Work out the finished part from the listing and answer in its coordinate system (mm). Face numbers are marked on the shaded views. A direction names the side the tool comes from. Round coordinates to 2 decimals unless told otherwise and drop trailing zeros. Loops run counter-clockwise (first coordinate to the right, second up) from the corner with the lowest first, then second, coordinate; pieces in that order, holes last. Notation, with made-up numbers: (67, -12.5) - (91, -12.5) arc R6 ccw to (91, -4.5) - close; hole circle Ø1 at (39, 32.25). An arc over 180 degrees is marked (long way). Return JSON: item names as keys, results as strings.
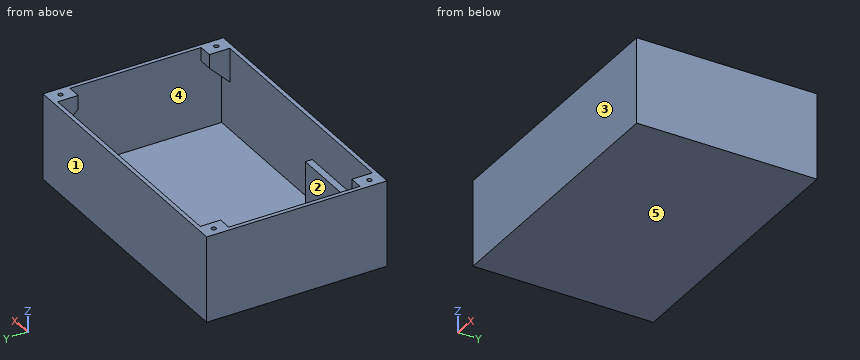
Autodesk Inventor part; units mm, degrees
ref_plane "YZ Plane" through (0, 0, 0) normal (1, 0, 0) x (0, 1, 0)
ref_plane "XZ Plane" through (0, 0, 0) normal (0, 1, 0) x (-1, 0, 0)
ref_plane "XY Plane" through (0, 0, 0) normal (0, 0, 1) x (1, 0, 0)
sketch "Sketch7" plane through (0, 0, 0) normal (0, 0, 1) x (1, 0, 0)
  line L0 (100.625, -66.125) -> (-100.625, -66.125)
  line L1 (-100.625, -66.125) -> (-100.625, 66.125)
  line L2 (-100.625, 66.125) -> (100.625, 66.125)
  line L3 (100.625, 66.125) -> (100.625, -66.125)
  line L4 (100.625, -66.125) -> (-100.625, 66.125) construction
  line L5 (-100.625, -66.125) -> (100.625, 66.125) construction
  point P0 (0, 0)
  dimension "d15" = 201.25
  dimension "d16" = 132.25
extrude "Box Outside" add sketch "Sketch7" along normal blind 63
sketch "Sketch8" plane through (0, 0, 63) normal (0, 0, 1) x (1, 0, 0)
  line L0 (-97.625, 63.125) -> (97.625, 63.125)
  line L1 (97.625, 63.125) -> (97.625, -63.125)
  line L2 (97.625, -63.125) -> (-97.625, -63.125)
  line L3 (-97.625, -63.125) -> (-97.625, 63.125)
  line L4 (100.625, 66.125) -> (-100.625, 66.125)
  line L5 (-100.625, 66.125) -> (-100.625, -66.125)
  line L6 (-100.625, -66.125) -> (100.625, -66.125)
  line L7 (100.625, -66.125) -> (100.625, 66.125)
  point P0 (0, 0)
  dimension "d19" = 3
  dimension "d20" = 3
  dimension "d21" = 3
  dimension "d22" = 3
extrude "Box Cut" cut sketch "Sketch8" against normal blind 60 contours L0 L1 L2 L3
sketch "Sketch9" plane through (-97.625, -63.125, 63) normal (0, 1, 0) x (1, 0, 0)
  line L0 (0, 0) -> (10, 0)
  line L1 (10, 0) -> (10, 25)
  line L2 (10, 25) -> (0, 25)
  line L3 (0, 25) -> (0, 0)
  point P0 (97.625, 63)
  dimension "d25" = 10
  dimension "d26" = 25
extrude "ScrewHole Box LB" add sketch "Sketch9" along normal blind 15
sketch "Sketch10" plane through (-97.625, -63.125, 3) normal (0, 1, 0) x (1, 0, 0)
  line L0 (195.25, -60) -> (195.25, 0)
  line L1 (195.25, -60) -> (185.25, -60)
  line L2 (185.25, -60) -> (185.25, -35)
  line L3 (185.25, -35) -> (195.25, -35)
  line L4 (195.25, -35) -> (195.25, -60)
  point P0 (97.625, 3)
  dimension "d29" = 10
  dimension "d30" = 25
extrude "ScrewHole Box RB" add sketch "Sketch10" along normal blind 15
sketch "Sketch11" plane through (-97.625, 63.125, 63) normal (0, -1, 0) x (1, 0, 0)
  line L0 (0, 0) -> (195.25, 0)
  line L1 (0, 0) -> (10, 0)
  line L2 (10, 0) -> (10, -25)
  line L3 (10, -25) -> (0, -25)
  line L4 (0, -25) -> (0, 0)
  point P0 (97.625, -63)
  dimension "d33" = 10
  dimension "d34" = 25
extrude "ScrewHole Box LU" add sketch "Sketch11" along normal blind 15
sketch "Sketch13" plane through (97.625, -63.125, 3) normal (-1, 0, 0) x (0, 0, 1)
  line L0 (60, 126.25) -> (0, 126.25)
  line L1 (60, 126.25) -> (35, 126.25)
  line L2 (35, 126.25) -> (35, 111.25)
  line L3 (35, 111.25) -> (60, 111.25)
  line L4 (60, 111.25) -> (60, 126.25)
  point P0 (-3, 63.125)
  dimension "d37" = 25
  dimension "d38" = 15
extrude "ScrewHole Box RU" add sketch "Sketch13" along normal blind 10
sketch "Sketch27" plane through (0, 0, 63) normal (0, 0, 1) x (1, 0, 0)
  line L0 (-87.625, -63.125) -> (-87.625, -48.125)
  line L1 (-100.625, 66.125) -> (-100.625, -66.125)
  line L2 (-87.625, -48.125) -> (-100.625, -48.125)
  line L3 (-100.625, -48.125) -> (-100.625, -66.125)
  line L4 (-100.625, -66.125) -> (-87.625, -66.125)
  line L5 (-87.625, -66.125) -> (-87.625, -48.125)
  line L6 (-87.625, -48.125) -> (-100.625, -66.125)
  line L7 (-87.625, -66.125) -> (-100.625, -48.125)
  circle A0 centre (-94.125, -57.125) radius 2.4
  point P0 (0, 0)
  dimension "d84" = 4.8
extrude "Outside ScrewHole LB" cut sketch "Sketch27" against normal blind 26 contours A0 L7 L6 | L6 L7 A0 | A0 L6 L7 | L7 L6 A0
sketch "Sketch29" plane through (0, 0, 63) normal (0, 0, 1) x (1, 0, 0)
  line L0 (-87.625, -63.125) -> (-87.625, -48.125)
  line L1 (-100.625, -66.125) -> (100.625, -66.125)
  line L2 (-87.625, -48.125) -> (-100.625, -48.125)
  line L3 (-100.625, -48.125) -> (-100.625, -66.125)
  line L4 (-100.625, -66.125) -> (-87.625, -66.125)
  line L5 (-87.625, -66.125) -> (-87.625, -48.125)
  line L6 (-87.625, -48.125) -> (-100.625, -66.125)
  circle A0 centre (-94.125, -57.125) radius 2.4
  point P0 (0, 0)
extrude "ScrewRibbon LB" add sketch "Sketch29" against normal blind 2 contours A0 L6 | L6 A0
sketch "Sketch30" plane through (0, 0, 63) normal (0, 0, 1) x (1, 0, 0)
  line L0 (-97.625, -48.125) -> (-87.625, -48.125)
  line L1 (-100.625, -66.125) -> (100.625, -66.125)
  line L2 (-87.625, -48.125) -> (-100.625, -48.125)
  line L3 (-100.625, -48.125) -> (-100.625, -66.125)
  line L4 (-100.625, -66.125) -> (-87.625, -66.125)
  line L5 (-87.625, -66.125) -> (-87.625, -48.125)
  line L6 (-87.625, -48.125) -> (-100.625, -66.125)
  circle A0 centre (-94.125, -57.125) radius 1.7
  point P0 (0, 0)
  dimension "d92" = 3.4
extrude "Inside ScrewHole LB" cut sketch "Sketch30" against normal blind 24 contours A0 L6 | L6 A0
sketch "Sketch31" plane through (0, 0, 63) normal (0, 0, 1) x (1, 0, 0)
  line L0 (-100.625, 66.125) -> (-100.625, -66.125)
  line L1 (-87.625, 48.125) -> (-97.625, 48.125)
  line L2 (-100.625, 66.125) -> (-87.625, 66.125)
  line L3 (-87.625, 66.125) -> (-87.625, 48.125)
  line L4 (-87.625, 48.125) -> (-100.625, 48.125)
  line L5 (-100.625, 48.125) -> (-100.625, 66.125)
  line L6 (-100.625, 66.125) -> (-87.625, 48.125)
  circle A0 centre (-94.125, 57.125) radius 2.4
  point P0 (0, 0)
  dimension "d95" = 4.8
extrude "Outside ScrewHole LU" cut sketch "Sketch31" against normal blind 24 contours A0 L6 | L6 A0
sketch "Sketch32" plane through (0, 0, 63) normal (0, 0, 1) x (1, 0, 0)
  line L0 (-97.625, 48.125) -> (-87.625, 48.125)
  line L1 (-100.625, 66.125) -> (-100.625, -66.125)
  line L2 (-87.625, 48.125) -> (-100.625, 48.125)
  line L3 (-100.625, 48.125) -> (-100.625, 66.125)
  line L4 (-100.625, 66.125) -> (-87.625, 66.125)
  line L5 (-87.625, 66.125) -> (-87.625, 48.125)
  line L6 (-87.625, 66.125) -> (-100.625, 48.125)
  circle A0 centre (-94.125, 57.125) radius 2.4
  point P0 (0, 0)
  dimension "d98" = 4.8
extrude "ScrewRibbon LU" add sketch "Sketch32" against normal blind 2 contours A0 L6 | L6 A0
sketch "Sketch33" plane through (0, 0, 63) normal (0, 0, 1) x (1, 0, 0)
  line L0 (100.625, 66.125) -> (-100.625, 66.125)
  line L1 (-87.625, 48.125) -> (-97.625, 48.125)
  line L2 (-100.625, 66.125) -> (-87.625, 66.125)
  line L3 (-87.625, 66.125) -> (-87.625, 48.125)
  line L4 (-87.625, 48.125) -> (-100.625, 48.125)
  line L5 (-100.625, 48.125) -> (-100.625, 66.125)
  line L6 (-100.625, 66.125) -> (-87.625, 48.125)
  circle A0 centre (-94.125, 57.125) radius 1.7
  point P0 (0, 0)
  dimension "d101" = 3.4
extrude "Inside ScrewHole LU" cut sketch "Sketch33" against normal blind 21.75 contours A0 L6 | L6 A0
sketch "Sketch34" plane through (0, 0, 63) normal (0, 0, 1) x (1, 0, 0)
  line L0 (87.625, 48.125) -> (87.625, 63.125)
  line L1 (100.625, 66.125) -> (-100.625, 66.125)
  line L2 (87.625, 48.125) -> (100.625, 48.125)
  line L3 (100.625, 48.125) -> (100.625, 66.125)
  line L4 (100.625, 66.125) -> (87.625, 66.125)
  line L5 (87.625, 66.125) -> (87.625, 48.125)
  line L6 (100.625, 66.125) -> (87.625, 48.125)
  circle A0 centre (94.125, 57.125) radius 2.4
  point P0 (0, 0)
  dimension "d104" = 4.8
extrude "Outside ScrewHole RU" cut sketch "Sketch34" against normal blind 37 contours A0 L6 | L6 A0
sketch "Sketch35" plane through (0, 0, 63) normal (0, 0, 1) x (1, 0, 0)
  line L0 (100.625, -66.125) -> (100.625, 66.125)
  line L1 (97.625, 48.125) -> (87.625, 48.125)
  line L2 (100.625, 66.125) -> (87.625, 66.125)
  line L3 (87.625, 66.125) -> (87.625, 48.125)
  line L4 (87.625, 48.125) -> (100.625, 48.125)
  line L5 (100.625, 48.125) -> (100.625, 66.125)
  line L6 (100.625, 66.125) -> (-100.625, 66.125)
  line L7 (100.625, 66.125) -> (87.625, 48.125)
  circle A0 centre (94.125, 57.125) radius 2.4
  point P0 (0, 0)
  dimension "d107" = 4.8
extrude "ScrewRibbon RU" add sketch "Sketch35" against normal blind 2 contours A0 L7 | L7 A0
sketch "Sketch36" plane through (0, 0, 63) normal (0, 0, 1) x (1, 0, 0)
  line L0 (97.625, 48.125) -> (87.625, 48.125)
  line L1 (100.625, -66.125) -> (100.625, 66.125)
  line L2 (87.625, 48.125) -> (100.625, 48.125)
  line L3 (100.625, 48.125) -> (100.625, 66.125)
  line L4 (100.625, 66.125) -> (87.625, 66.125)
  line L5 (87.625, 66.125) -> (87.625, 48.125)
  line L6 (87.625, 48.125) -> (100.625, 66.125)
  circle A0 centre (94.125, 57.125) radius 2.4
  circle A1 centre (94.125, 57.125) radius 1.7
  point P0 (0, 0)
  dimension "d110" = 3.4
extrude "Inside ScrewHole RU" cut sketch "Sketch36" against normal blind 20 contours A1 L6 | L6 A1
sketch "Sketch37" plane through (0, 0, 63) normal (0, 0, 1) x (1, 0, 0)
  line L0 (100.625, -66.125) -> (100.625, 66.125)
  line L1 (87.625, -63.125) -> (87.625, -48.125)
  line L2 (100.625, -66.125) -> (87.625, -66.125)
  line L3 (87.625, -66.125) -> (87.625, -48.125)
  line L4 (87.625, -48.125) -> (100.625, -48.125)
  line L5 (100.625, -48.125) -> (100.625, -66.125)
  line L6 (87.625, -66.125) -> (100.625, -48.125)
  circle A0 centre (94.125, -57.125) radius 2.4
  point P0 (0, 0)
  dimension "d113" = 4.8
extrude "Outside ScrewHole RB" cut sketch "Sketch37" against normal blind 27.5 contours A0 L6 | L6 A0
sketch "Sketch38" plane through (0, 0, 63) normal (0, 0, 1) x (1, 0, 0)
  line L0 (97.625, -48.125) -> (87.625, -48.125)
  line L1 (100.625, -66.125) -> (100.625, 66.125)
  line L2 (87.625, -48.125) -> (100.625, -48.125)
  line L3 (100.625, -48.125) -> (100.625, -66.125)
  line L4 (100.625, -66.125) -> (87.625, -66.125)
  line L5 (87.625, -66.125) -> (87.625, -48.125)
  line L6 (100.625, -48.125) -> (87.625, -66.125)
  circle A0 centre (94.125, -57.125) radius 2.4
  point P0 (0, 0)
  dimension "d116" = 4.8
extrude "ScrewRibbon RB" add sketch "Sketch38" against normal blind 2 contours A0 L6 | L6 A0
sketch "Sketch39" plane through (0, 0, 63) normal (0, 0, 1) x (1, 0, 0)
  line L0 (87.625, -63.125) -> (87.625, -48.125)
  line L1 (100.625, -66.125) -> (100.625, 66.125)
  line L2 (87.625, -48.125) -> (100.625, -48.125)
  line L3 (100.625, -48.125) -> (100.625, -66.125)
  line L4 (100.625, -66.125) -> (87.625, -66.125)
  line L5 (87.625, -66.125) -> (87.625, -48.125)
  line L6 (87.625, -66.125) -> (100.625, -48.125)
  circle A0 centre (94.125, -57.125) radius 2.4
  circle A1 centre (94.125, -57.125) radius 1.7
  point P0 (0, 0)
  dimension "d119" = 3.4
extrude "Inside ScrewHole RB" cut sketch "Sketch39" against normal blind 20 contours A1 L6 | L6 A1
sketch "Sketch42" plane through (-97.625, -63.125, 3) normal (0, 1, 0) x (1, 0, 0)
  line L0 (195.25, 0) -> (0, 0)
  line L1 (30, 0) -> (84, 0)
  line L2 (84, 0) -> (84, -31)
  line L3 (84, -31) -> (30, -31)
  line L4 (30, -31) -> (30, 0)
  line L5 (0, -35) -> (0, 0)
  line L6 (195.25, -35) -> (195.25, 0)
  point P0 (97.625, 3)
  dimension "d134" = 54
  dimension "d135" = 31
  dimension "d197" = 111.25
extrude "ESPHolder" add sketch "Sketch42" along normal blind 5
chamfer "Chamfer1" distance 15 angle 45 1 edges at (-92.625, -48.125, 38)
chamfer "Chamfer2" distance 15 angle 45 1 edges at (-92.625, 48.125, 38)
chamfer "Chamfer3" distance 15 angle 45 1 edges at (92.625, 48.125, 38)
chamfer "Chamfer4" distance 15 angle 45 1 edges at (92.625, -48.125, 38)
properties part number "Box2"
1) Find the intervals of material crossed by L1, parallel to Y at x = -53, z = 26 (3 decimals); L2, parallel to X at y = 39, z = 32 (3 decimals); L3, parallel to Y at x = 79.5, z = 17 (3 decimals), in increasing order.
Verdict:
{"L1": "y = -66.125 to -58.125, 63.125 to 66.125", "L2": "x = -100.625 to -97.625, 97.625 to 100.625", "L3": "y = -66.125 to -63.125, 63.125 to 66.125"}
2) Section B-B (x = 58.5) is taken. Give the vertices of the cut face in (y, z) (3 decimals), and give its area (3 significant figures).
Verdict:
{"outline": "(-66.125, 0) - (66.125, 0) - (66.125, 63) - (63.125, 63) - (63.125, 3) - (-63.125, 3) - (-63.125, 63) - (-66.125, 63) - close", "area": "757 mm2"}
3) A tool of negligible diameter and unlimited length cuts with its end or side. For the marked faces 1 and 2, from which of +Z, -Z, +X, -X, +Y, -Y can it reach the whole face along a straight path? Write none if from no direction.
Verdict:
{"face 1": "+Z, -Z, +X, -X, +Y", "face 2": "+Z"}
4) Determine the mould class of the marked faces 3, 4 and 5 for opening direction Z: pulls with the +Z half, pulls with the -Z half, needs draft (parallel to the pull), parting line crosses it, or undercut.
Verdict:
{"face 3": "needs draft", "face 4": "undercut", "face 5": "pulls with the -Z half"}
5) Section A-A (z = 12) is taken. Give the vertices of the cut face in (x, y) (3 decimals), and give its area (4 significant figures).
Verdict:
{"outline": "(-100.625, -66.125) - (100.625, -66.125) - (100.625, 66.125) - (-100.625, 66.125) - close; hole (-97.625, -63.125) - (-67.625, -63.125) - (-67.625, -58.125) - (-13.625, -58.125) - (-13.625, -63.125) - (97.625, -63.125) - (97.625, 63.125) - (-97.625, 63.125) - close", "area": "2,235 mm2"}
6) Flat-ended cylindrical pins translate along their axes: pin 1 (8 mm diameter, centred on x = 10.5, y = 12.5, fed in from -Z); pin 2 (3 mm diameter, centred on x = -3, y = 27, fed in from +Z). Find the tip coordinate at first contact, or state that the pin passes through.
Verdict:
{"pin 1": "stops at z = 0", "pin 2": "stops at z = 3"}
7) Section D-D (z = 48.5) is taken. Give the vertices of the cut face in (x, y) (3 decimals).
Verdict:
{"outline": "(-100.625, -66.125) - (100.625, -66.125) - (100.625, 66.125) - (-100.625, 66.125) - close; hole (-97.625, -52.625) - (-87.625, -52.625) - (-87.625, -63.125) - (87.625, -63.125) - (87.625, -52.625) - (97.625, -52.625) - (97.625, 52.625) - (87.625, 52.625) - (87.625, 63.125) - (-87.625, 63.125) - (-87.625, 52.625) - (-97.625, 52.625) - close; hole circle Ø4.8 at (-94.125, -57.125); hole circle Ø4.8 at (-94.125, 57.125); hole circle Ø4.8 at (94.125, -57.125); hole circle Ø4.8 at (94.125, 57.125)"}
8) Section C-C (y = 0.5) is taken. Give the vertices of the cut face in (x, z) (3 decimals).
Verdict:
{"outline": "(-100.625, 0) - (100.625, 0) - (100.625, 63) - (97.625, 63) - (97.625, 3) - (-97.625, 3) - (-97.625, 63) - (-100.625, 63) - close"}
